Verification items for the finished model (mm, model axes). Face numbers are marked on the shaded views. A direction names the side the tool comes from. Coordinates: 2 decimals unless noted, no trailing zeros. Loops run counter-clockwise (first coordinate to the right, second up) from the corner with the lowest first, then second, coordinate; pieces in that order, holes last. Notation, with made-up numbers: (31.5, 4.5) - (79.5, 4.5) arc R29 ccw to (79.5, 33.5) - close; hole circle Ø7 at (66, -29.75). An arc over 180 degrees is marked (long way). Answer as CSV lines item,"result". Start each with the question number.
1. Cross-section at D-D (z = -131). Enter the section's corners in (x, y), plus the area to 3 significant figures.
2. Cross-section at A-A (z = -83). Enter the section's corners in (x, y), plus the area to 3 significant figures.
3. Gauge pin test, flat ends, axial feed: P1, Ø3, axis at x = -7, y = 5, coming from the +Z side; P2, Ø2, axis at x = 37.5, y = 1.5, coming from the +Z side; P3, Ø2.5, axis at x = -36, y = 14, coming from the -Z side. Record the tip position at first contact, or that the pin passes through.
4. Cross-section at C-C (x = 46). Enter the section's corners in (y, z).
5. Release check for a two-part mould opening along X. For the marked faces 3, 4 and 5 record: pulls with the +X half, pulls with the -X half, needs draft (parallel to the pull), parting line crosses it, or undercut.
6. Cross-section at B-B (x = 19). Enter the section's corners in (y, z).
7. Set-up check for the marked faces 1 and 2: record each of +Z, -Z, +X, -X, +Y, -Y from which the full face is reachable in a straight line by a thin tool's end or side.
8. Material ranges on line 1 (X direction, y = 3.5, z = -84); line 2 (Z direction, x = -20.5, y = 12.25); line 3 (Z direction, x = -34.5, y = 5.75), recorded low to high. Write a range as [from, to].
```python
from build123d import *

# Parameters (mm, degrees)
BOSS_EXTRUDE1_DEPTH = 16
CUT_EXTRUDE1_DEPTH  = 9.2
CUT_EXTRUDE2_REACH  = 152.177
SKETCH3_W           = 70
SKETCH3_H           = 50
SKETCH7_OUTSIDE_W   = 133.782
SKETCH7_OUTSIDE_H   = 99.382
CUT_EXTRUDE5_DEPTH  = 4
BOSS_EXTRUDE3_START = -12
BOSS_EXTRUDE3_DEPTH = 12
CUT_EXTRUDE7_REACH  = 174.842
SKETCH9_R           = 38
CUT_EXTRUDE8_REACH  = 174.842
SKETCH10_R          = 38
FILLET1_R           = 5
SKETCH12_W          = 25
SKETCH12_H          = 3.5
CUT_EXTRUDE10_DEPTH = 4
SKETCH13_W          = 3.5
SKETCH13_H          = 3.5
CUT_EXTRUDE11_DEPTH = 1.5
CUT_EXTRUDE12_REACH = 157.926
SKETCH14_W          = 70
SKETCH14_H          = 2
CUT_EXTRUDE13_DEPTH = 4


with BuildPart() as part:
    # Sketch1 → Boss-Extrude1 (new body)
    with BuildSketch(Plane(origin=(0, 0, 0), x_dir=(1, 0, 0), z_dir=(0, 1, 0))):
        with BuildLine():
            Line((-53, 129.147822281), (-53, 80))
            Line((-53, 80), (-41, 68))
            Line((-41, 68), (41, 68))
            Line((41, 68), (53, 80))
            Line((53, 80), (53, 129.147822281))
            ThreePointArc((53, 129.147822281), (0, 139.6), (-53, 129.147822281))
        make_face()
    extrude(amount=BOSS_EXTRUDE1_DEPTH)

    # Sketch2 → Cut-Extrude1 (cut)
    with BuildSketch(Plane.XZ):
        Polygon((-33.8, -122.965685425), (-33.8, -62.4), (35, -62.4), (35, -122.965685425), (24.765685425, -133.2), (-23.565685425, -133.2), align=None)
    extrude(amount=-CUT_EXTRUDE1_DEPTH, mode=Mode.SUBTRACT)

    # Sketch3 → Cut-Extrude2 (cut, up to next)
    with BuildSketch(Plane(origin=(0, 16, 0), x_dir=(1, 0, 0), z_dir=(0, 1, 0)), mode=Mode.PRIVATE) as cut_extrude2_sk1:
        with Locations((0, 100)):
            Rectangle(SKETCH3_W, SKETCH3_H)
    cut_extrude2_tool1 = extrude(cut_extrude2_sk1.sketch, amount=-CUT_EXTRUDE2_REACH, mode=Mode.PRIVATE) & part.part
    add(cut_extrude2_tool1.solids().sort_by_distance((0, 16, -100))[0], mode=Mode.SUBTRACT)

    # Sketch7 outside → Cut-Extrude5 (cut)
    with BuildSketch(Plane.XZ):
        with Locations((0, -103.8)):
            Rectangle(SKETCH7_OUTSIDE_W, SKETCH7_OUTSIDE_H)
        with BuildLine():
            Line((-50, -81.242640687), (-50, -127.120258024))
            ThreePointArc((-50, -127.120258024), (0, -136.6), (50, -127.120258024))
            Line((50, -127.120258024), (50, -81.242640687))
            Line((50, -81.242640687), (39.757359313, -71))
            Line((39.757359313, -71), (35, -71))
            Line((35, -71), (-33.8, -71))
            Line((-33.8, -71), (-39.757359313, -71))
            Line((-39.757359313, -71), (-50, -81.242640687))
        make_face(mode=Mode.SUBTRACT)
    extrude(amount=-CUT_EXTRUDE5_DEPTH, mode=Mode.SUBTRACT)

    # Sketch8 → Boss-Extrude3 (add)
    with BuildSketch(Plane(origin=(0, 16, 0), x_dir=(1, 0, 0), z_dir=(0, 1, 0)).offset(BOSS_EXTRUDE3_START)):
        with BuildLine():
            Line((70.810563619, 120.308038302), (53, 102.497474683))
            Line((53, 102.497474683), (53, 129.147822281))
            ThreePointArc((53, 129.147822281), (62.062866201, 125.045434299), (70.810563619, 120.308038302))
        make_face()
    boss_extrude3 = extrude(amount=BOSS_EXTRUDE3_DEPTH)

    # Mirror1: Boss-Extrude3 across plane
    add(boss_extrude3.mirror(Plane(origin=(0, 0, 0), x_dir=(0, 0, 1), z_dir=(1, 0, 0))))

    # Cut-Extrude7: up to this plane
    cut_extrude7_end = Plane(origin=(53, 16, -80), z_dir=(-1, 0, 0))
    # Sketch9 → Cut-Extrude7 (cut, up to the surface)
    with BuildSketch(Plane(origin=(95.55930096, 0, -95.55930096), x_dir=(0, 1, 0), z_dir=(-0.7071067811865488, 0, 0.7071067811865464)), mode=Mode.PRIVATE) as cut_extrude7_sk1:
        Circle(SKETCH9_R)
    cut_extrude7_tool1 = split(extrude(cut_extrude7_sk1.sketch, amount=CUT_EXTRUDE7_REACH, mode=Mode.PRIVATE), bisect_by=cut_extrude7_end, keep=Keep.BOTH, mode=Mode.PRIVATE)
    add(cut_extrude7_tool1.solids().sort_by_distance((95.559301, 0, -95.559301))[0], mode=Mode.SUBTRACT)

    # Cut-Extrude8: up to this plane
    cut_extrude8_end = Plane(origin=(-53, 16, -129.147822281), z_dir=(1, 0, 0))
    # Sketch10 → Cut-Extrude8 (cut, up to the surface)
    with BuildSketch(Plane(origin=(-95.55930096, 0, -95.55930096), x_dir=(0, 1, 0), z_dir=(0.7071067811865488, 0, 0.7071067811865464)), mode=Mode.PRIVATE) as cut_extrude8_sk1:
        Circle(SKETCH10_R)
    cut_extrude8_tool1 = split(extrude(cut_extrude8_sk1.sketch, amount=CUT_EXTRUDE8_REACH, mode=Mode.PRIVATE), bisect_by=cut_extrude8_end, keep=Keep.BOTH, mode=Mode.PRIVATE)
    add(cut_extrude8_tool1.solids().sort_by_distance((-95.559301, 0, -95.559301))[0], mode=Mode.SUBTRACT)

    # Fillet1
    fillet1_edges = [part.edges().sort_by_distance(p)[0] for p in [
        (70.810563619, 15.399324293, -120.308038302),
        (69.207065384, 9.508661419, -121.237544106),
        (-70.810563619, 15.399324293, -120.308038302),
        (-69.207065384, 9.508661419, -121.237544106),
    ]]
    fillet(fillet1_edges, radius=FILLET1_R)

    # Sketch12 → Cut-Extrude10 (cut)
    with BuildSketch(Plane(origin=(0, 16, 0), x_dir=(1, 0, 0), z_dir=(0, 1, 0))):
        with Locations((0, 73.25)):
            Rectangle(SKETCH12_W, SKETCH12_H)
    extrude(amount=-CUT_EXTRUDE10_DEPTH, mode=Mode.SUBTRACT)

    # Sketch13 → Cut-Extrude11 (cut)
    with BuildSketch(Plane(origin=(0, 16, 0), x_dir=(1, 0, 0), z_dir=(0, 1, 0))):
        with Locations((-14.25, 73.25)):
            Rectangle(SKETCH13_W, SKETCH13_H)
        with Locations((14.25, 73.25)):
            Rectangle(SKETCH13_W, SKETCH13_H)
    extrude(amount=-CUT_EXTRUDE11_DEPTH, mode=Mode.SUBTRACT)

    # Sketch14 → Cut-Extrude12 (cut, up to next)
    with BuildSketch(Plane(origin=(0, 16, 0), x_dir=(1, 0, 0), z_dir=(0, 1, 0)), mode=Mode.PRIVATE) as cut_extrude12_sk1:
        with Locations((0, 69)):
            Rectangle(SKETCH14_W, SKETCH14_H)
    cut_extrude12_tool1 = extrude(cut_extrude12_sk1.sketch, amount=-CUT_EXTRUDE12_REACH, mode=Mode.PRIVATE) & part.part
    add(cut_extrude12_tool1.solids().sort_by_distance((0, 16, -69))[0], mode=Mode.SUBTRACT)

    # Sketch15 → Cut-Extrude13 (cut)
    with BuildSketch(Plane(origin=(0, 16, 0), x_dir=(1, 0, 0), z_dir=(0, 1, 0))):
        Polygon((-35, 77.6), (-35, 125), (35, 125), (35, 77.6), (38.4, 77.6), (38.4, 128.4), (-38.4, 128.4), (-38.4, 77.6), align=None)
    extrude(amount=-CUT_EXTRUDE13_DEPTH, mode=Mode.SUBTRACT)


solid = part.part
```
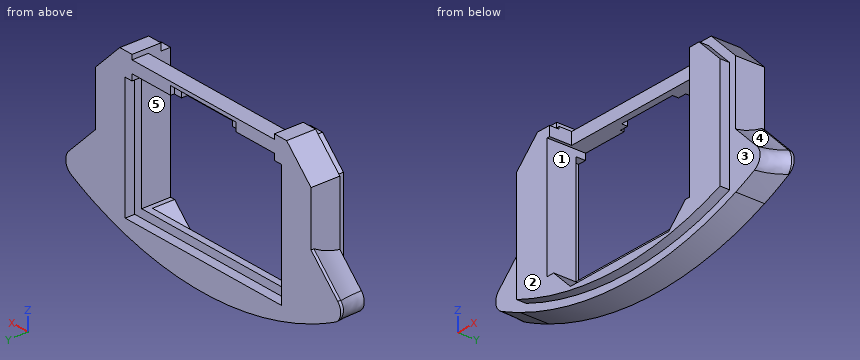
Values follow:
1,outline,"(-48.24, 4) - (-38.71, 4) - (-38.71, 0) - (-25.77, 0) - (-25.77, 9.2) - (26.97, 9.2) - (26.97, 0) - (38.71, 0) - (38.71, 4) - (48.24, 4) - (48.24, 16) - (-48.24, 16) - close"
1,area,"982 mm²"
2,outline,"(-53, 4) - (-50, 4) - (-50, 0) - (-35, 0) - (-35, 12) - (-38.4, 12) - (-38.4, 16) - (-53, 16) - close; (35, 0) - (50, 0) - (50, 4) - (53, 4) - (53, 16) - (38.4, 16) - (38.4, 12) - (35, 12) - close"
2,area,"525 mm²"
3,P1,"stops at z = -133.2"
3,P2,"stops at z = -71"
3,P3,"stops at z = -135.21"
4,outline,"(0, -128.62) - (4, -128.62) - (4, -131.8) - (16, -131.8) - (16, -73) - (4, -73) - (4, -77.24) - (0, -77.24) - close"
5,face 3,"needs draft"
5,face 4,"pulls with the +X half"
5,face 5,"undercut"
6,outline,"(0, -135.27) - (4, -135.27) - (4, -138.3) - (16, -138.3) - (16, -128.4) - (12, -128.4) - (12, -125) - (9.2, -125) - (9.2, -133.2) - (0, -133.2) - close; (9.2, -75) - (16, -75) - (16, -70) - (9.2, -70) - close"
7,face 1,"+Y, -Y"
7,face 2,"+Z, -Z, +X, -X, -Y"
8,line 1,"x = [-50, -35], [35, 50]"
8,line 2,"z = [-138.09, -128.4], [-75, -70]"
8,line 3,"z = [-135.27, -125], [-75, -70]"
